Model file for the job. Use its own axes, mm. Give positions to 0.01 mm unless a question says otherwise; leave off trailing zeros. Loops run counter-clockwise (first coordinate to the right, second up) from the corner with the lowest first, then second, coordinate; pieces in that order, holes last. Notation, with made-up numbers: (74, -8) -> (129, -8) arc R13 ccw to (129, 12) -> close; hole circle Ø8 at (20.25, 37). An arc over 180 degrees is marked (long way). Use CSV: the item, a comma, the result in double quotes. Start each with the question number.
(1) Cut at C-C on x = 17. Write the cut outline in (y, z).
(2) Cut at A-A on z = -8.89. Write the cut outline in (x, y).
(3) Drill centre lines: probe 1 along X at (y, z) = (0.5, -8.89); probe 2 along Z at (x, y) = (-16, 1.75); probe 3 along X at (y, z) = (1.7, 8.5). Where is each one in solid material? Low to high.
(4) Cut at B-B on y = 0.5. Write the cut outline in (x, z), then the cut area to 3 significant figures.
(5) Flat gauge pins, fed straight in: pin 1 (0.9 mm diameter, centred on y = 1, z = -1, fed in from -X); pin 2 (2.5 mm diameter, centred on x = 16.51, z = -8.89, fed in from +Y). Where does each tip first touch, or does it go through?
from build123d import *

# Parameters (mm, degrees)
CROQUIS1_R              = 1.5
SALIENTE_EXTRUIR1_DEPTH = 1.8


with BuildPart() as part:
    # Croquis1 → Saliente-Extruir1 (new body)
    with BuildSketch(Plane(origin=(0, 0, 0), x_dir=(1, 0, 0), z_dir=(0, 1, 0))):
        with BuildLine():
            Line((-13.97, 11.43), (-16.51, 11.43))
            ThreePointArc((-16.51, 11.43), (-19.05, 8.89), (-16.51, 6.35))
            Line((-16.51, 6.35), (-13.97, 6.35))
            Line((-13.97, 6.35), (-13.97, -6.35))
            Line((-13.97, -6.35), (-16.51, -6.35))
            ThreePointArc((-16.51, -6.35), (-19.05, -8.89), (-16.51, -11.43))
            Line((-16.51, -11.43), (-13.97, -11.43))
            Line((-13.97, -11.43), (13.97, -11.43))
            Line((13.97, -11.43), (16.51, -11.43))
            ThreePointArc((16.51, -11.43), (19.05, -8.89), (16.51, -6.35))
            Line((16.51, -6.35), (13.97, -6.35))
            Line((13.97, -6.35), (13.97, 6.35))
            Line((13.97, 6.35), (16.51, 6.35))
            ThreePointArc((16.51, 6.35), (19.05, 8.89), (16.51, 11.43))
            Line((16.51, 11.43), (13.97, 11.43))
            Line((13.97, 11.43), (-13.97, 11.43))
        make_face()
        with Locations(Location((-16.51, 8.89, 0), (0, 0, 270))):
            Circle(CROQUIS1_R, mode=Mode.SUBTRACT)
        with Locations(Location((16.51, 8.89, 0), (0, 0, 90))):
            Circle(CROQUIS1_R, mode=Mode.SUBTRACT)
        with Locations(Location((16.51, -8.89, 0), (0, 0, 270))):
            Circle(CROQUIS1_R, mode=Mode.SUBTRACT)
        with Locations(Location((-16.51, -8.89, 0), (0, 0, 90))):
            Circle(CROQUIS1_R, mode=Mode.SUBTRACT)
    extrude(amount=SALIENTE_EXTRUIR1_DEPTH)


solid = part.part
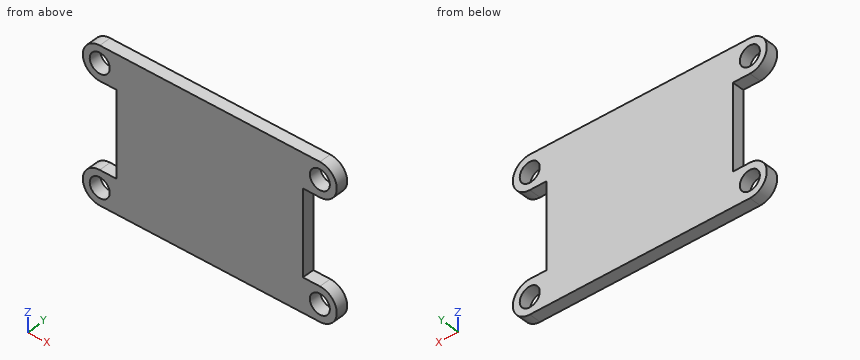
Check result:
1,outline,"(0, -11.38) -> (1.8, -11.38) -> (1.8, -10.31) -> (0, -10.31) -> close; (0, -7.47) -> (1.8, -7.47) -> (1.8, -6.4) -> (0, -6.4) -> close; (0, 6.4) -> (1.8, 6.4) -> (1.8, 7.47) -> (0, 7.47) -> close; (0, 10.31) -> (1.8, 10.31) -> (1.8, 11.38) -> (0, 11.38) -> close"
2,outline,"(-19.05, 0) -> (-18.01, 0) -> (-18.01, 1.8) -> (-19.05, 1.8) -> close; (-15.01, 0) -> (15.01, 0) -> (15.01, 1.8) -> (-15.01, 1.8) -> close; (18.01, 0) -> (19.05, 0) -> (19.05, 1.8) -> (18.01, 1.8) -> close"
3,probe 1,"-19.05 to -18.01, -15.01 to 15.01, 18.01 to 19.05"
3,probe 2,"-11.43 to -10.3, -7.48 to -6.35, 6.35 to 7.48, 10.3 to 11.43"
3,probe 3,"-19.02 to -17.96, -15.06 to 15.06, 17.96 to 19.02"
4,outline,"(-16.51, -11.43) -> (16.51, -11.43) arc R2.54 ccw to (16.51, -6.35) -> (13.97, -6.35) -> (13.97, 6.35) -> (16.51, 6.35) arc R2.54 ccw to (16.51, 11.43) -> (-16.51, 11.43) arc R2.54 ccw to (-16.51, 6.35) -> (-13.97, 6.35) -> (-13.97, -6.35) -> (-16.51, -6.35) arc R2.54 ccw to start; hole circle Ø3 at (-16.51, -8.89); hole circle Ø3 at (-16.51, 8.89); hole circle Ø3 at (16.51, -8.89); hole circle Ø3 at (16.51, 8.89)"
4,area,"703 mm²"
5,pin 1,"x = -13.97"
5,pin 2,"through"
